Autodesk Inventor part; units mm, degrees
ref_plane "Work Plane1" through (1.525, 0, 0) normal (0, 0, 1) x (1, 0, 0)
ref_plane "YZ Plane" through (0, 0, 0) normal (1, 0, 0) x (0, 1, 0)
ref_plane "XZ Plane" through (0, 0, 0) normal (0, 1, 0) x (-1, 0, 0)
sketch "Sketch1" plane through (0, 0, 0) normal (0, 0, 1) x (1, 0, 0)
  line L0 (0, 8.7) -> (0, 6)
  line L1 (70, 6) -> (100, 6)
  line L2 (100, 6) -> (100, 0)
  line L3 (100, 0) -> (-0.6001, 0)
  line L4 (-20.7201, 0) -> (120.12, 0)
  line L5 (-0.6001, 0) -> (-0.6001, 8.7)
  line L6 (-0.6001, 8.7) -> (0, 8.7)
  line L7 (70, 6) -> (68.9264, 6)
  line L8 (68.9264, 6) -> (0, 6)
  line L9 (0, -1.74) -> (0, 10.44)
  dimension "d0" = 100
  dimension "d1" = 30
  dimension "d2" = 12
  dimension "d9" = 0.6001
  dimension "d10" = 17.4
  dimension "d13" = 1.0736
  dimension "d14" = 12
revolve "Body" add sketch "Sketch1" angle 360 about axis through (100, 0, 0) along (-1, 0, 0)
sketch "Sketch2" plane through (-0.6001, 0, 0) normal (-1, 0, 0) x (0, 0, 1)
  line L0 (0, 10.9697) -> (9.5, 5.4848)
  line L1 (9.5, 5.4848) -> (9.5, -5.4848)
  line L2 (9.5, -5.4848) -> (0, -10.9697)
  line L3 (0, -10.9697) -> (-9.5, -5.4848)
  line L4 (-9.5, -5.4848) -> (-9.5, 5.4848)
  line L5 (-9.5, 5.4848) -> (0, 10.9697)
  point P0 (0, 0)
  point P1 (0, 0)
  dimension "d11" = 19
extrude "Head" add sketch "Sketch2" along normal blind 6.9
sketch "Sketch4" plane through (0, 0, 0) normal (0, 0, 1) x (1, 0, 0)
  line L0 (-7.5001, 9.5) -> (-7.5001, 10.9697)
  line L1 (-7.5001, 10.9697) -> (-6.6516, 10.9697)
  line L2 (-6.6516, 10.9697) -> (-7.5001, 9.5)
  line L3 (-8.8801, 0) -> (0.7799, 0)
  line L4 (-0.6001, 10.9697) -> (-7.5001, 10.9697)
  line L5 (-7.5001, 5.4848) -> (-7.5001, 10.9697)
  dimension "d5" = 30
  dimension "d19" = 19
revolve "Chamfer1" cut sketch "Sketch4" angle 360 about axis through (-10, 0, 0) along (1, 0, 0)
thread "Thread"
chamfer "Chamfer2" distance 1.0735 distance2 1.0736 1 edges at (100, -6, 0) measured on face at (100, 1.8579, -1.646)
ref_plane "Work Plane1" through (1.525, 0, 0) normal (0, 0, 1) x (1, 0, 0)
equation "\"d0\" = NLG"
equation "\"d1\" = GEL"
equation "\"d2\" = GD"
equation "\"d10\" = SD2"
equation "\"d14\" = BDM"
equation "\"d11\" = SW"
equation "\"d3\" = KOH - SD"
equation "\"d5\" = ANG1"
equation "\"d19\" = SW0"
equation "\"d15\" = GEL"
equation "\"d6\" = -0.5 * SPD + 0.5 * GD"
equation "\"NLG\" = 100"
equation "\"GD\" = NND"
equation "\"BDM\" = NND"
equation "\"KOH\" = 7.5"
equation "\"GEL\" = 30"
equation "\"SW\" = 19"
equation "\"SW0\" = SW"
equation "\"SPD\" = NND - 1.2269 * PTC"
equation "\"SD2\" = 17.4"
equation "\"SD\" = 0.6"
equation "\"ANG1\" = 30deg"
equation "\"GAL\" = 0.61345 * PTC"
equation "\"GUL\" = 0.61345 * PTC"
equation "\"RR\" = 0.6"
equation "\"GD1\" = THREADDIA - 1.2269 * PTC"
equation "\"THREADDIA\" = 12"
equation "\"TOA\" = 30deg"
equation "\"PTC\" = 1.75"
equation "\"NND\" = 12"
equation "\"E0\" = 1.155 * SW"
properties part number "DIN 931-1 - M12 x 100" material "Steel, Mild"
Geometry check sheet. Reference: the model listing, model coordinates, mm. A direction names the side the tool comes from. Give positions to 0.01 mm unless a question says otherwise; leave off trailing zeros. Loops run counter-clockwise (first coordinate to the right, second up) from the corner with the lowest first, then second, coordinate; pieces in that order, holes last. Notation, with made-up numbers: (87.25, 22.5) -> (143.25, 22.5) arc R22 ccw to (143.25, 55.5) -> close; hole circle Ø11 at (-1.75, 29). An arc over 180 degrees is marked (long way). Answer in a Markdown table with one row per item. Add a question column.
1) Gauge pin test, flat ends, axial feed: P1, Ø1.5, axis at y = 0.5, z = 7, coming from the +X side; P2, Ø3, axis at x = 24.5, z = 0, coming from the +Y side; P3, Ø4, axis at x = 66, y = 3.5, coming from the -Z side. Record the tip position at first contact, or that the pin passes through.
2) Set-up check for faces 1 (the face through (-0.296, -1.886, -8.493)), 2 (the face through (-4, 8.2, -4.8)): record each of +Z, -Z, +X, -X, +Y, -Y from which the full face is reachable in a straight line by a thin tool's end or side.
3) Material ranges on probe 1 along X at (y, z) = (-7.75, 4.5); probe 2 along X at (y, z) = (6.5, 1.5); probe 3 along Y at (x, z) = (56.5, -0.5), recorded low to high. Write a range as from..to.
4) Cross-section at A-A on x = 15.5. Record the boundary of the cut face in (y, z).
Outcome:
| question | item | result |
|---|---|---|
| 1 | P1 | stops at x = 0 |
| 1 | P2 | stops at y = 6 |
| 1 | P3 | stops at z = -5.81 |
| 2 | face 1 | +X |
| 2 | face 2 | -Z, +X, -X, +Y |
| 3 | probe 1 | x = -7.5..-0.6 |
| 3 | probe 2 | x = -7.5..0 |
| 3 | probe 3 | y = -5.98..5.98 |
| 4 | outline | circle Ø12 at (0, 0) |
